Autodesk Inventor part; units mm, degrees
ref_plane "YZ Plane" through (0, 0, 0) normal (1, 0, 0) x (0, 1, 0)
ref_plane "XZ Plane" through (0, 0, 0) normal (0, 1, 0) x (-1, 0, 0)
ref_plane "XY Plane" through (0, 0, 0) normal (0, 0, 1) x (1, 0, 0)
sketch "Sketch1" plane through (0, 0, 0) normal (0, 0, 1) x (1, 0, 0)
  circle A0 centre (0, 0) radius 3.175
  dimension "d0" = 6.35
extrude "Extrusion1" add sketch "Sketch1" along normal blind 15.875
sketch "Sketch2" plane through (0, 0, 0) normal (0, 0, -1) x (-1, 0, 0)
  circle A0 centre (0, 0) radius 3.175
  circle A1 centre (0, 0) radius 4.7625
  dimension "d3" = 9.525
extrude "Extrusion2" add sketch "Sketch2" along normal blind 6.35 contours A0 | A1
sketch "Sketch3" plane through (0, 0, -6.35) normal (0, 0, -1) x (-1, 0, 0)
  circle A0 centre (0, 0) radius 4.7625
  line L0 (-1.3748, 2.3812) -> (1.3748, 2.3813)
  line L1 (1.3748, 2.3813) -> (2.7496, 0)
  line L2 (2.7496, 0) -> (1.3748, -2.3812)
  line L3 (1.3748, -2.3812) -> (-1.3748, -2.3812)
  line L4 (-1.3748, -2.3812) -> (-2.7496, 0)
  line L5 (-2.7496, 0) -> (-1.3748, 2.3812)
  dimension "d6" = 4.7625
extrude "Extrusion3" cut sketch "Sketch3" against normal blind 3.175 contours L0 L1 L2 L3 L4 L5
chamfer "Chamfer1" distance 0.508 angle 45 3 edges at (-3.175, 0, 15.875) (4.7625, 0, 0) (4.7625, 0, -6.35)
thread "Thread1"
properties part number "14-20 x750" material "Steel"
Geometry check sheet. Reference: the model listing, model coordinates, mm. A direction names the side the tool comes from. Round coordinates to 2 decimals unless told otherwise and drop trailing zeros. Order: outer loops, then holes, each group sorted by start corner. A loop starts at its lowest first (then second) coordinate and runs counter-clockwise, first axis right, second up. Notation, with made-up numbers: M -4.5,81 L 43.5,81 A18 ccw 43.5,90 Z; hole C 4,22 d10. An arc over 180 degrees is marked long. Answer in a Markdown table with one row per item.
(1) Tool access check on faces 4 (the face through (0, 0, 15.875)), 5 (the face through (2, -3, 0)), 6 (the face through (2.05, -1.21, -4.78)). Record the directions out of +Z, -Z, +X, -X, +Y, -Y that give a thin tool (end or side, any length) a straight path to the whole face; none if there is none.
Responses:
| item | result |
|---|---|
| face 4 | +Z, +X, -X, +Y, -Y |
| face 5 | +Z |
| face 6 | -Z |
(2) Draft check along Y on faces 1 (the face through (0, -2.381, -5)), 2 (the face through (-2, -2, -6.35)), 3 (the face through (3.78, 2.9, -3.14)). Enter one of: released by +Y, released by -Y, zero draft, split by the parting line, or undercut.
Responses:
| item | result |
|---|---|
| face 1 | undercut |
| face 2 | zero draft |
| face 3 | split by the parting line |
(3) Go/stop test with flat-tipped pins: P1, Ø2.5, axis at x = 0, y = 1, coming from the -Z side (3 decimals); P2, Ø2, axis at x = 0.5, z = -4.5, coming from the +Y side; P3, Ø1, axis at y = -3, z = 13, coming from the -X side; P4, Ø2, axis at x = -4, z = -1, coming from the -Y side. Record where each tip stops, or that it passes through.
Responses:
| item | result |
|---|---|
| P1 | stops at z = -3.175 |
| P2 | stops at y = 4.76 |
| P3 | stops at x = -1.96 |
| P4 | stops at y = -3.7 |
(4) Scan lines: probe 1 along Z at (x, y) = (1.25, 3.5); probe 2 along Y at (x, z) = (0, 3.5) (3 decimals); probe 3 along Z at (x, y) = (1, -1.25) (3 decimals). Record each from-to range of solid material in increasing order. Write a range as from..to.
Responses:
| item | result |
|---|---|
| probe 1 | z = -6.35..0 |
| probe 2 | y = -3.175..3.175 |
| probe 3 | z = -3.175..15.875 |
(5) Sectioned sample at B-B, the plane z = 6.5. Record the cut outline in (x, y) (3 decimals), and give its area (3 significant figures).
Responses:
| item | result |
|---|---|
| outline | C 0,0 d6.35 |
| area | 31.7 mm² |
